```python
from build123d import *

# Parameters (mm, degrees)
BASE_FLANGE1_DEPTH           = 1.6002
EDGE_FLANGE1_STRIP_W         = 8.0264
EDGE_FLANGE1_STRIP_H         = 1.6002
EDGE_FLANGE1_STRIP_CUT_DEPTH = 176.239897552
EDGE_FLANGE1_DEPTH           = 176.239897552
EDGE_FLANGE2_STRIP_W         = 8.0264
EDGE_FLANGE2_STRIP_H         = 1.6002
EDGE_FLANGE2_STRIP_CUT_DEPTH = 89.864191945
EDGE_FLANGE2_DEPTH           = 89.864191945
EDGE_FLANGE3_STRIP_W         = 8.0264
EDGE_FLANGE3_STRIP_H         = 1.6002
EDGE_FLANGE3_STRIP_CUT_DEPTH = 238.716677062
EDGE_FLANGE3_DEPTH           = 238.716677062
SKETCH18_R                   = 2.7051
CUT_EXTRUDE3_DEPTH           = 7.62
SKETCH19_R                   = 2.7051
CUT_EXTRUDE4_DEPTH           = 7.62
SKETCH20_R                   = 2.7051
CUT_EXTRUDE5_DEPTH           = 7.62


# Read off the part's stored shape, not the designer's step: Base-Flange1
# Sheet-metal steps are written as plain solids
with BuildPart() as part:
    # Base-Flange1 outline → Base-Flange1 (new body)
    with BuildSketch(Plane(origin=(0, 0, 0), x_dir=(1, 0, 0), z_dir=(0, 0, -1))):
        with BuildLine():
            Line((0, 0), (-66.675, 0))
            Line((-66.675, 0), (-66.675, -1.5748))
            Line((-66.675, -1.5748), (-69.85, -1.5748))
            Line((-69.85, -1.5748), (-69.85, -240.291477062))
            Line((-69.85, -240.291477062), (-66.802, -240.291477062))
            Line((-66.802, -240.291477062), (-64.646738531, -242.446738531))
            Line((-64.646738531, -242.446738531), (-1.103159021, -178.903159021))
            Line((-1.103159021, -178.903159021), (-2.899210245, -177.107107796))
            ThreePointArc((-2.899210245, -177.107107796), (-3.009330803, -176.553494368), (-2.54, -176.239897552))
            Line((-2.54, -176.239897552), (0, -176.239897552))
            Line((0, -176.239897552), (0, 0))
        make_face()
    extrude(amount=BASE_FLANGE1_DEPTH)

    # Edge-Flange1 strip (across the edge) → Edge-Flange1 strip cut (cut)
    with BuildSketch(Plane(origin=(0, 176.239897552, -1.6002), x_dir=(-1, 0, 0), z_dir=(0, -1, 0))):
        with Locations((-1.6002, -0.8001)):
            Rectangle(EDGE_FLANGE1_STRIP_W, EDGE_FLANGE1_STRIP_H)
    extrude(amount=EDGE_FLANGE1_STRIP_CUT_DEPTH, mode=Mode.SUBTRACT)

    # Edge-Flange1 section (across the edge) → Edge-Flange1 (add)
    with BuildSketch(Plane(origin=(0, 176.239897552, -1.6002), x_dir=(-1, 0, 0), z_dir=(0, -1, 0))):
        with BuildLine():
            Line((0, 0.8128), (0, 17.4498))
            Line((0, 17.4498), (1.6002, 17.4498))
            Line((1.6002, 17.4498), (1.6002, 0.8128))
            ThreePointArc((1.6002, 0.8128), (1.838263608, 0.238063608), (2.413, 0))
            Line((2.413, 0), (2.413, -1.6002))
            ThreePointArc((2.413, -1.6002), (0.706751337, -0.893448663), (0, 0.8128))
        make_face()
    extrude(amount=EDGE_FLANGE1_DEPTH)

    # Edge-Flange2 strip (across the edge) → Edge-Flange2 strip cut (cut)
    with BuildSketch(Plane(origin=(-64.646738531, 242.446738531, -1.6002), x_dir=(-0.7071067811865479, -0.7071067811865472, -3.58046925441613e-15), z_dir=(0.7071067811865472, -0.7071067811865479, 0))):
        with Locations((-1.6002, -0.8001)):
            Rectangle(EDGE_FLANGE2_STRIP_W, EDGE_FLANGE2_STRIP_H)
    extrude(amount=EDGE_FLANGE2_STRIP_CUT_DEPTH, mode=Mode.SUBTRACT)

    # Edge-Flange2 section (across the edge) → Edge-Flange2 (add)
    with BuildSketch(Plane(origin=(-64.646738531, 242.446738531, -1.6002), x_dir=(-0.7071067811865479, -0.7071067811865472, -3.58046925441613e-15), z_dir=(0.7071067811865472, -0.7071067811865479, 0))):
        with BuildLine():
            Line((0, 0.8128), (0, 17.4498))
            Line((0, 17.4498), (1.6002, 17.4498))
            Line((1.6002, 17.4498), (1.6002, 0.8128))
            ThreePointArc((1.6002, 0.8128), (1.838263608, 0.238063608), (2.413, 0))
            Line((2.413, 0), (2.413, -1.6002))
            ThreePointArc((2.413, -1.6002), (0.706751337, -0.893448663), (0, 0.8128))
        make_face()
    extrude(amount=EDGE_FLANGE2_DEPTH)

    # Edge-Flange3 strip (across the edge) → Edge-Flange3 strip cut (cut)
    with BuildSketch(Plane(origin=(-69.85, 240.291477062, 0), x_dir=(1, 0, 0), z_dir=(0, -1, 0))):
        with Locations((-1.6002, -0.8001)):
            Rectangle(EDGE_FLANGE3_STRIP_W, EDGE_FLANGE3_STRIP_H)
    extrude(amount=EDGE_FLANGE3_STRIP_CUT_DEPTH, mode=Mode.SUBTRACT)

    # Edge-Flange3 section (across the edge) → Edge-Flange3 (add)
    with BuildSketch(Plane(origin=(-69.85, 240.291477062, 0), x_dir=(1, 0, 0), z_dir=(0, -1, 0))):
        with BuildLine():
            Line((0, 0.8128), (0, 17.4498))
            Line((0, 17.4498), (1.6002, 17.4498))
            Line((1.6002, 17.4498), (1.6002, 0.8128))
            ThreePointArc((1.6002, 0.8128), (1.838263608, 0.238063608), (2.413, 0))
            Line((2.413, 0), (2.413, -1.6002))
            ThreePointArc((2.413, -1.6002), (0.706751337, -0.893448663), (0, 0.8128))
        make_face()
    extrude(amount=EDGE_FLANGE3_DEPTH)

    # Sketch18 → Cut-Extrude3 (cut)
    with BuildSketch(Plane(origin=(0, 0, 0), x_dir=(0, 0, -1), z_dir=(1, 0, 0))):
        with Locations((11.1252, 38.1)):
            Circle(SKETCH18_R)
        with Locations((11.1252, 139.7)):
            Circle(SKETCH18_R)
    extrude(amount=-CUT_EXTRUDE3_DEPTH, mode=Mode.SUBTRACT)

    # Sketch19 → Cut-Extrude4 (cut)
    with BuildSketch(Plane(origin=(88.9, 88.9, 0), x_dir=(0, 0, -1), z_dir=(0.7071067811865517, 0.7071067811865434, 3.37416286723297e-15))):
        with Locations(Location((11.1252, 176.523585695, 0), (0, 0, 90))):
            Circle(SKETCH19_R)
    extrude(amount=-CUT_EXTRUDE4_DEPTH, mode=Mode.SUBTRACT)

    # Sketch20 → Cut-Extrude5 (cut)
    with BuildSketch(Plane.ZY.offset(69.85)):
        with Locations((9.525, 25.4)):
            Circle(SKETCH20_R)
        with Locations((9.525, 114.3)):
            Circle(SKETCH20_R)
        with Locations((9.525, 203.2)):
            Circle(SKETCH20_R)
    extrude(amount=-CUT_EXTRUDE5_DEPTH, mode=Mode.SUBTRACT)


solid = part.part
```
Part model, mm, in its own coordinate system. A direction names the side the tool comes from. Give positions to 0.01 mm unless a question says otherwise; leave off trailing zeros. Loops run counter-clockwise (first coordinate to the right, second up) from the corner with the lowest first, then second, coordinate; pieces in that order, holes last. Notation, with made-up numbers: M -24,1.5 L -10,1.5 A23 ccw -10,40.5 Z; hole C -28.75,14.5 d5. An arc over 180 degrees is marked long. Return JSON: item names as keys, results as strings.
1) Pull direction Z, two halves, no side cores. Call faces 1 (the face through (-0.789, 39.928, -9.131)), 2 (the face through (-33.83, 210.61, -0.69)), 3 (the face through (-34, 211, -19.05)): released by +Z, released by -Z, zero draft, split by the parting line, or undercut.
Calculated:
{"face 1": "undercut", "face 2": "released by +Z", "face 3": "released by -Z"}
2) Drill centre lines: line 1 (X direction, y = 98, z = -14); line 2 (X direction, y = 186, z = 9.5). Where is each one in solid material? Low to high.
Calculated:
{"line 1": "x = -1.6 to 0", "line 2": "x = -69.85 to -68.25"}
3) Saw through at A-A, the plane y = 25.4. List the corners of the cut face in (x, z).
Calculated:
{"outline": "M -69.85,0.81 A2.41 ccw -67.44,-1.6 L -2.41,-1.6 A0.81 cw -1.6,-2.41 L -1.6,-19.05 L 0,-19.05 L 0,-2.41 A2.41 ccw -2.41,0 L -67.44,0 A0.81 cw -68.25,0.81 L -68.25,6.82 L -69.85,6.82 Z; M -69.85,12.23 L -68.25,12.23 L -68.25,17.45 L -69.85,17.45 Z"}
4) Flat gauge pins, fed straight in: pin 1 Ø2.5 at (x, z) = (-68.5, 3) entering from +Y; pin 2 Ø5 at (y, z) = (150, 13) entering from +X; pin 3 Ø1.6 at (x, z) = (-68.5, 9.5) entering from -Y. Where does each tip first touch, or does it go through?
Calculated:
{"pin 1": "stops at y = 240.29", "pin 2": "stops at x = -68.25", "pin 3": "stops at y = 1.57"}
5) 3-axis set-ups, long thin cutter, end or side, ignore diameter. For faces 4 (the face through (-1.6, 89, -11)), 5 (the face through (-68.25, 123, 9)), 6 (the face through (-38.246, 214.93, -12.161)): which of +Z, -Z, +X, -X, +Y, -Y reach the whole face in a straight line?
Calculated:
{"face 4": "-Z, -X, -Y", "face 5": "+Z, +X, +Y, -Y", "face 6": "none"}
